Autodesk Inventor part; units mm, degrees
ref_plane "YZ Plane" through (0, 0, 0) normal (1, 0, 0) x (0, 1, 0)
ref_plane "XZ Plane" through (0, 0, 0) normal (0, 1, 0) x (-1, 0, 0)
ref_plane "XY Plane" through (0, 0, 0) normal (0, 0, 1) x (1, 0, 0)
sketch "Sketch1" plane through (0, 0, 0) normal (0, 1, 0) x (-1, 0, 0)
  circle A0 centre (0, 0) radius 2
  dimension "d0" = 4
extrude "Extrusion1" add sketch "Sketch1" along normal blind 30
chamfer "Chamfer1" distance 1 angle 45 1 edges at (2, 0, 0)
chamfer "Chamfer2" distance 1 angle 45 1 edges at (2, 30, 0)
properties part number "thread"
The model under review builds one solid part; all positions refer to its coordinate system, in mm. Give positions to 0.01 mm unless a question says otherwise; leave off trailing zeros. Order: outer loops, then holes, each group sorted by start corner. A loop starts at its lowest first (then second) coordinate and runs counter-clockwise, first axis right, second up. Notation, with made-up numbers: M 54.5,69.25 L 112.5,69.25 A24 ccw 112.5,89.25 Z; hole C 46.5,-35.75 d2. An arc over 180 degrees is marked long. Answer in a Markdown table with one row per item. Add a question column.
1. To check wall thickness, follow line 1 along X through (y, z) = (25, 0.1); line 2 along Z through (x, y) = (-0.15, 7.75); line 3 along X through (y, z) = (19.75, -1.3). State the ranges of each line that lie inside material, in increasing order.
2. Add section C-C on y = 27. State the section outline as (x, z) points, plus the area to 3 significant figures.
3. For pin 1 Ø1 at (x, z) = (1, -1) entering from +Y; pin 2 Ø1.5 at (y, z) = (24.5, 1) entering from -X; pin 3 Ø2 at (y, z) = (6.5, 1.5) entering from -X, all flat-tipped, find the tip position at first contact; note any pin that passes through.
4. Add section B-B on x = 0. State the section outline as (y, z) points.
5. Add section A-A on z = 0. State the section outline as (x, y) points, plus the area to 3 significant figures.
The answers:
| question | item | result |
|---|---|---|
| 1 | line 1 | -2 to 2 |
| 1 | line 2 | -1.99 to 1.99 |
| 1 | line 3 | -1.52 to 1.52 |
| 2 | outline | C 0,0 d4 |
| 2 | area | 12.6 mm2 |
| 3 | pin 1 | y = 30 |
| 3 | pin 2 | x = -1.98 |
| 3 | pin 3 | x = -1.94 |
| 4 | outline | M 0,-1 L 1,-2 L 29,-2 L 30,-1 L 30,1 L 29,2 L 1,2 L 0,1 Z |
| 5 | outline | M -2,1 L -1,0 L 1,0 L 2,1 L 2,29 L 1,30 L -1,30 L -2,29 Z |
| 5 | area | 118 mm2 |
